For this review, use the dimensioned drawing (mm, ordinates from the lowest corner) and the shaded views. A direction names the side the tool comes from. Round coordinates to 2 decimals unless told otherwise and drop trailing zeros. Write each loop counter-clockwise with the first axis right and the second up, starting at its lowest first coordinate (ties: lowest second). Pieces come first, ordered by that corner, then holes. Notation, with made-up numbers: M 77,38.5 L 84,38.5 A15 cw 84,56.5 Z; hole C 49,-3 d2. An arc over 180 degrees is marked long. Use one line per item in the form item = value. Start each with the question number.
Item 1: Add section D-D (z = 4.1). State the section outline as (x, y) points (1 decimal), and give its area (3 significant figures).
Item 2: For the marked faces 1 and 2, list the 3-axis set-ups (+Z, -Z, +X, -X, +Y, -Y) from which the entire face can be reached by the end or side of a thin tool; tool diameter is ignored.
Item 3: Add section A-A (z = 0.95). State the section outline as (x, y) points.
Item 4: For line 1 (Z direction, x = 4.75, y = 8.5); line 2 (Y direction, x = 8, z = 3.25); line 3 (Y direction, x = 2, z = 4.25) (1 decimal), list the stretches that pass through material, from the lowest coordinate up. Write a range as [from, to].
Item 5: Draft analysis for pull direction Y (two halves, no side actions). For the marked faces 3, 4 and 5, state which applies: released by +Y, released by -Y, zero draft, split by the parting line, or undercut.
Item 6: Add section B-B (y = 8). State the section outline as (x, z) points.
Item 7: Add section C-C (x = 7.75). State the section outline as (y, z) points.
Item 8: For P1, Ø1.5, axis at y = 7, z = 4, coming from the +X side (1 decimal), flat-tipped, find the tip position at first contact; note if it passes through.
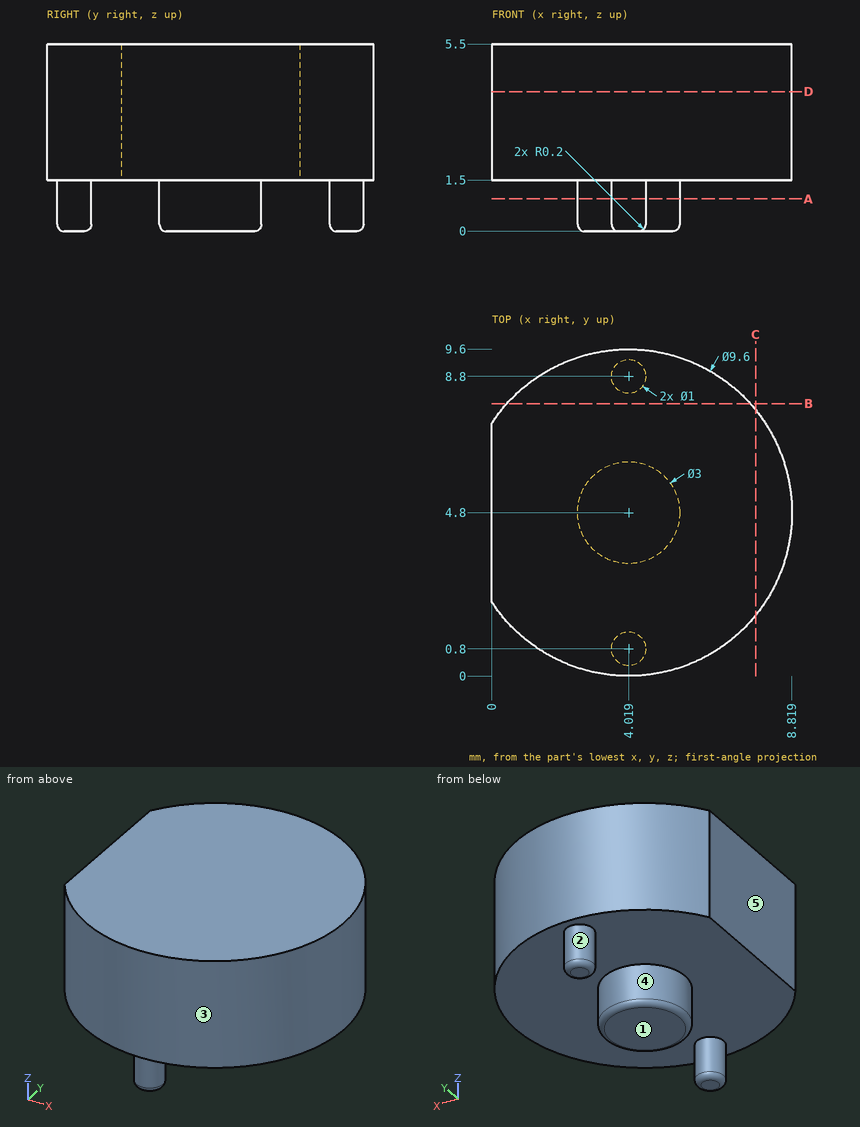
Calculated:
q1.outline = M 0,2.2 A4.8 ccw long 0,7.4 Z
q1.area = 69.6 mm^2
q2.face_1 = -Z, +X, -X, +Y, -Y
q2.face_2 = -Z
q3.outline = C 4.02,4.8 d3; C 4.02,0.8 d1; C 4.02,8.8 d1
q4.line_1 = [1.5, 5.5]
q4.line_2 = [2.12, 7.48]
q4.line_3 = [0.4, 9.2]
q5.face_3 = split by the parting line
q5.face_4 = undercut
q5.face_5 = zero draft
q6.outline = M 0.44,1.5 L 7.6,1.5 L 7.6,5.5 L 0.44,5.5 Z
q7.outline = M 1.78,1.5 L 7.82,1.5 L 7.82,5.5 L 1.78,5.5 Z
q8.P1 = 8.6
